Can you work these out from the drawing? Everything is in mm from the part's minimum corner. Give positions to 0.01 mm unless a question says otherwise; leave off trailing zeros. Order: outer loops, then holes, each group sorted by start corner. A loop starts at its lowest first (then second) coordinate and runs counter-clockwise, first axis right, second up. Notation, with made-up numbers: (49.25, -23.75) -> (57.25, -23.75) arc R32 ccw to (57.25, 2.25) -> close; hole circle Ø7 at (21, 63). An arc over 180 degrees is marked (long way). One line per item, written item: value.
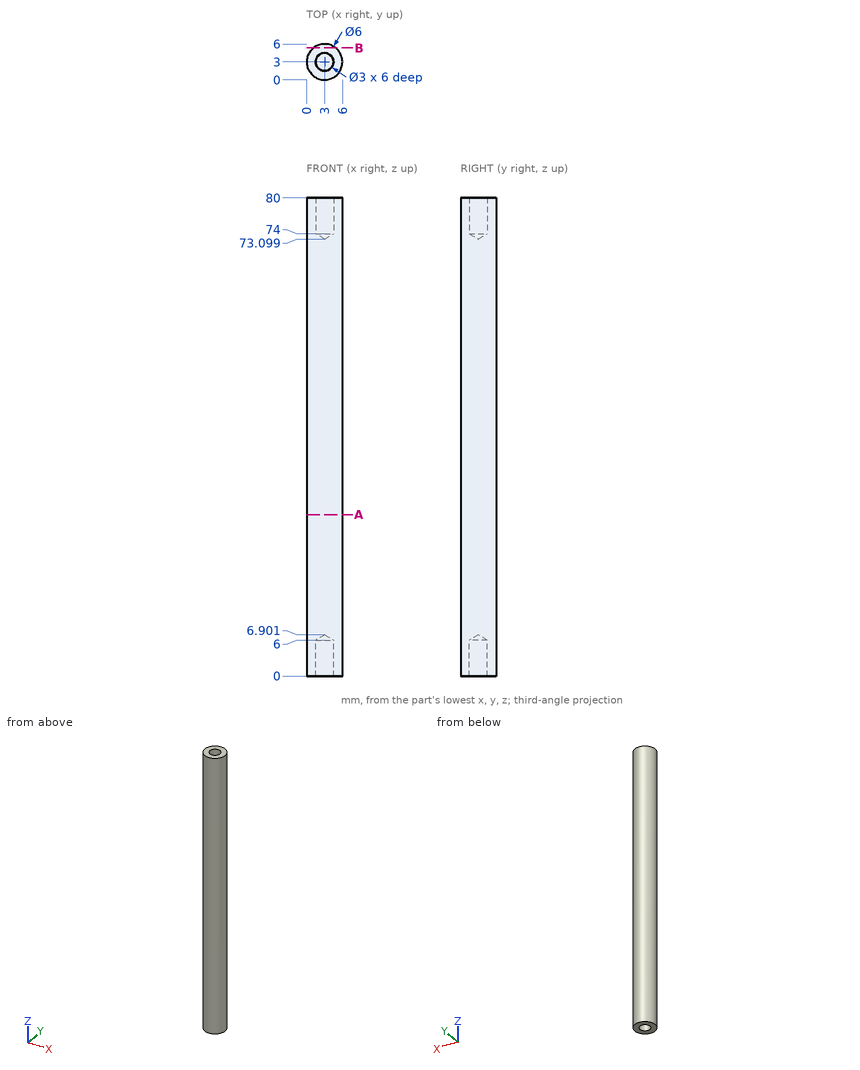
1) For P1, Ø2.5, axis at x = 3, y = 3, coming from the +Z side; P2, Ø1.5, axis at x = 2, y = 3.5, coming from the -Z side; P3, Ø1.5, axis at x = 4.5, z = 27.5, coming from the -Y side (1 decimal); P4, Ø1.8, axis at x = 3, y = 3, coming from the +Z side, each with a flat end and sliding along its axis, tell me the tip position at first contact or that it passes through.
Answer below:
P1: stops at z = 73.85
P2: stops at z = 0
P3: stops at y = 0.1
P4: stops at z = 73.64
2) If I drill on line 1 along Y through (x, z) = (3, 2.05); line 2 along Y through (x, z) = (3.15, 23.5); line 3 along Y through (x, z) = (3.9, 5), over which ranges is the centre line in solid material (lowest first)?
Answer below:
line 1: y = 0 to 1.5, 4.5 to 6
line 2: y = 0 to 6
line 3: y = 0.14 to 1.8, 4.2 to 5.86
3) Suppose I cut it at A-A, the plane z = 27. Write out the boundary of the cut face in (x, y), then the cut area to 3 significant figures.
Answer below:
outline: circle Ø6 at (3, 3)
area: 28.3 mm2
4) Suppose I cut it at B-B, the plane y = 5.35. Write out the boundary of the cut face in (x, z) (1 decimal).
Answer below:
outline: (1.1, 0) -> (4.9, 0) -> (4.9, 80) -> (1.1, 80) -> close
